Answer from the drawing. Dimensions are ordinates in mm from the lowest x, y and z of the part. A direction names the side the tool comes from. Coordinates: 2 decimals unless noted, no trailing zeros. Order: outer loops, then holes, each group sorted by start corner. A loop starts at its lowest first (then second) coordinate and runs counter-clockwise, first axis right, second up.
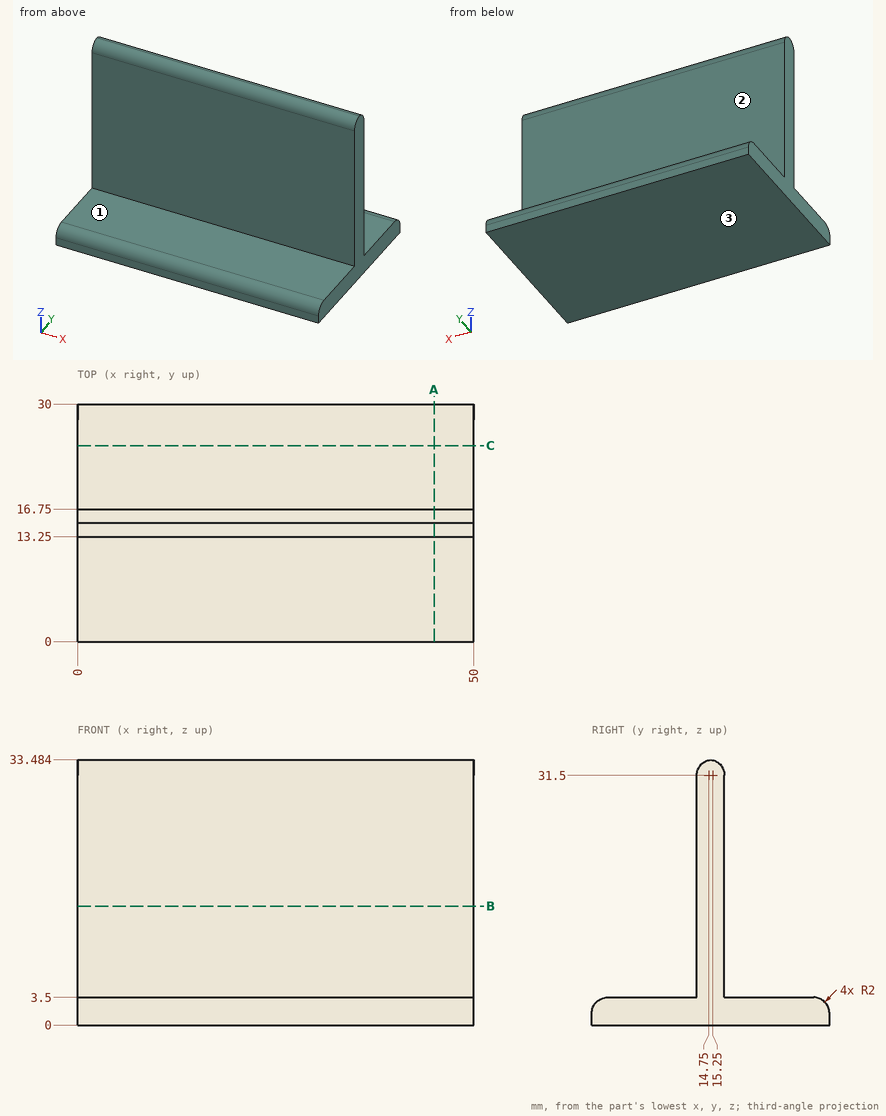
1. Consider probe 1 along Y at (x, z) = (42, 6); probe 2 along Z at (x, y) = (8, 21.25); probe 3 along Z at (x, y) = (19, 28.75) (1 decimal). Determine where each line is inside the solid, lowest interval first.
2. The part is cut by section B-B (z = 15). Determine the outline of the cut face in (x, y), plus the area to 3 significant figures.
3. The part is cut by section A-A (x = 45). Determine the outline of the cut face in (y, z).
4. For the marked faces 1, 2 and 3, determine the directions among +Z, -Z, +X, -X, +Y, -Y from which every point of the face is accessible in a straight line to the end or side of a thin tool.
5. The part is cut by section C-C (y = 24.75). Determine the outline of the cut face in (x, z), plus the area to 3 significant figures.
6. Flat-ended cylindrical pins translate along their axes: pin 1 (1.5 mm diameter, centred on x = 34, z = 23.5, fed in from +Y); pin 2 (1.5 mm diameter, centred on x = 35.5, z = 30, fed in from -Y); pin 3 (12.5 mm diameter, centred on x = 14.5, y = 24, fed in from +Z). Find the tip coordinate at first contact, or state that the pin passes through.
Worked out:
1. probe 1: y = 13.25 to 16.75
1. probe 2: z = 0 to 3.5
1. probe 3: z = 0 to 3.4
2. outline: (0, 13.25) - (50, 13.25) - (50, 16.75) - (0, 16.75) - close
2. area: 175 mm2
3. outline: (0, 0) - (30, 0) - (30, 1.5) arc R2 ccw to (28, 3.5) - (16.75, 3.5) - (16.75, 31.5) arc R2 ccw to (15, 33.48) arc R2 ccw to (13.25, 31.5) - (13.25, 3.5) - (2, 3.5) arc R2 ccw to (0, 1.5) - close
4. face 1: +Z, +X, -X, -Y
4. face 2: +Z, +X, -X, +Y
4. face 3: -Z, +X, -X, +Y, -Y
5. outline: (0, 0) - (50, 0) - (50, 3.5) - (0, 3.5) - close
5. area: 175 mm2
6. pin 1: stops at y = 16.75
6. pin 2: stops at y = 13.25
6. pin 3: stops at z = 3.5
